Here's the drawing with two shaded views (mm, measured from the low corner). I have some questions. Give positions to 0.01 mm unless a question says otherwise; leave off trailing zeros. Loops run counter-clockwise (first coordinate to the right, second up) from the corner with the lowest first, then second, coordinate; pieces in that order, holes last. Notation, with made-up numbers: (31.25, 52.25) -> (36.25, 52.25) arc R21 ccw to (36.25, 82.25) -> close; hole circle Ø4 at (73.5, -16.5). An arc over 180 degrees is marked (long way). Answer in a Markdown table with one row per item. Add a question column.
Item 1: For P1, Ø8, axis at x = 19, y = 116.5, coming from the +Z side; P2, Ø10, axis at x = 40, y = 28.5, coming from the +Z side (1 decimal); P3, Ø3, axis at x = 30.16, z = 6.35, coming from the +Y side; P4, Ø1.5, axis at y = 90, z = 19, coming from the -X side (1 decimal), each with a flat end and sliding along its axis, tell me the tip position at first contact or that it passes through.
Item 2: If I drill on line 1 (Y direction, x = 3, z = 27.5); line 2 (Z direction, x = 42.5, y = 134) (1 decimal); line 3 (Z direction, x = 21, y = 42.5) (1 decimal), over which ranges is the centre line in solid material (lowest first)?
Item 3: We'd pull the mould along X, two halves only. Please class the marked faces 1, 2 and 3: released by +X, released by -X, zero draft, split by the parting line, or undercut.
Item 4: If we section it at D-D (z = 26.5): Write out the boundary of the cut face in (x, y).
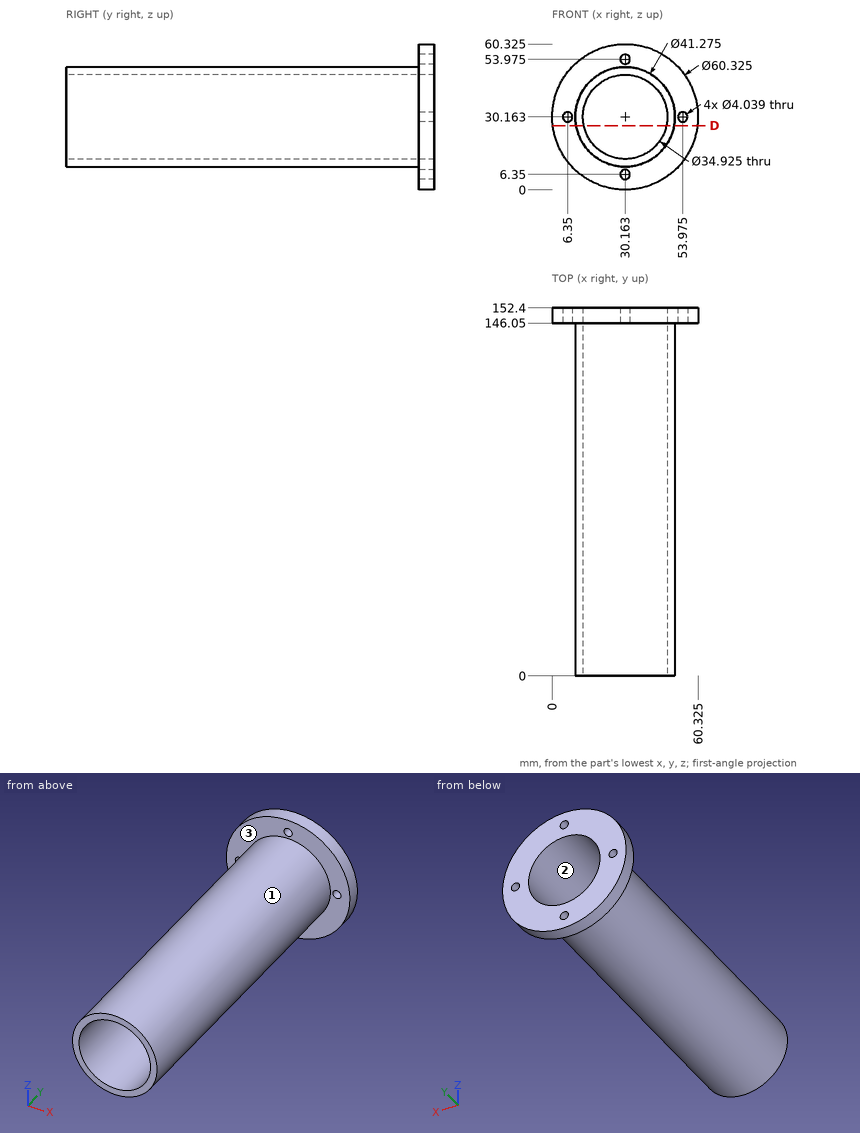
Recorded:
| question | item | result |
|---|---|---|
| 1 | P1 | stops at z = 49.52 |
| 1 | P2 | stops at z = 50.2 |
| 1 | P3 | passes through |
| 1 | P4 | stops at x = 12.3 |
| 2 | line 1 | y = 146.05 to 152.4 |
| 2 | line 2 | z = 13.6 to 17.8, 42.5 to 46.7 |
| 2 | line 3 | z = 11.7 to 15.3, 45 to 48.7 |
| 3 | face 1 | split by the parting line |
| 3 | face 2 | undercut |
| 3 | face 3 | zero draft |
| 4 | outline | (0.22, 146.05) -> (9.85, 146.05) -> (9.85, 0) -> (13.09, 0) -> (13.09, 152.4) -> (0.22, 152.4) -> close; (47.24, 0) -> (50.47, 0) -> (50.47, 146.05) -> (60.1, 146.05) -> (60.1, 152.4) -> (47.24, 152.4) -> close |
